Autodesk Inventor part; units mm, degrees
ref_plane "YZ Plane" through (0, 0, 0) normal (1, 0, 0) x (0, 1, 0)
ref_plane "XZ Plane" through (0, 0, 0) normal (0, 1, 0) x (-1, 0, 0)
ref_plane "XY Plane" through (0, 0, 0) normal (0, 0, 1) x (1, 0, 0)
sketch "Sketch1" plane through (0, 0, 0) normal (0, 0, 1) x (1, 0, 0)
  line L0 (0, 27) -> (138, 27)
  line L1 (138, 27) -> (138, 0)
  line L2 (138, 0) -> (138, -27)
  line L3 (138, -27) -> (27, -93) construction
  line L4 (27, -93) -> (0, -93)
  line L5 (0, -93) -> (0, 27) construction
  line L6 (0, 0) -> (138, 0) construction
  line L7 (0, 27) -> (-138, 27)
  line L8 (-138, 27) -> (-138, 0)
  line L9 (-138, 0) -> (-138, -27)
  line L10 (-138, -27) -> (-27, -93) construction
  line L11 (-27, -93) -> (0, -93)
  line L12 (27, -93) -> (138, -93)
  line L13 (138, -93) -> (138, -27)
  line L14 (-27, -93) -> (-138, -93)
  line L15 (-138, -93) -> (-138, -27)
  dimension "d0" = 138
  dimension "d2" = 27
  dimension "d3" = 54
  dimension "d4" = 27
  dimension "d5" = 120
extrude "Extrusion1" add sketch "Sketch1" along normal mid plane 60
sketch "Sketch2" plane through (-27, -93, 30) normal (0, -1, 0) x (1, 0, 0)
  circle A0 centre (27, -30) radius 24.5
  dimension "d20" = 49
extrude "Extrusion2" add sketch "Sketch2" along normal blind 51
sketch "Sketch3" plane through (-138, 27, 30) normal (0, 1, 0) x (1, 0, 0)
  circle A0 centre (138, 30) radius 10
  dimension "d12" = 20
extrude "Extrusion3" cut sketch "Sketch3" against normal through all
sketch "Sketch4" plane through (138, -27, 30) normal (1, 0, 0) x (0, 0, -1)
  circle A0 centre (30, 27) radius 10
  dimension "d16" = 20
extrude "Extrusion4" cut sketch "Sketch4" against normal through all
move or copy body "Move Body1" bodies to move or copy 1 copy no rotation origin (0, 0, 0) rotation axis (1, 0, 0) rotation angle 90
move or copy body "Move Body2" bodies to move or copy 1 copy no rotation origin (0, 0, 0) rotation axis (0, 0, 1) rotation angle 90
move or copy body "Move Body4" bodies to move or copy 1 copy no translate (0, 0, 144)
properties part number "UpperTorso_v2"
Input: part model. Units: mm. Frame: model coordinates. A direction names the side the tool comes from. Coordinates: 2 decimals unless noted, no trailing zeros. Write each loop counter-clockwise with the first axis right and the second up, starting at its lowest first coordinate (ties: lowest second). Pieces come first, ordered by that corner, then holes. Notation, with made-up numbers: (-34, 36) - (-7, 36) arc R15 cw to (-7, 57) - close; hole circle Ø4 at (-29, -30.75). An arc over 180 degrees is marked (long way). Put each result on its own line as item: value. Start each with the question number.
1) Ray query, L1, parallel to X at y = 0, z = 79; L2, parallel to Y at x = 0, z = 161.5; L3, parallel to Z at x = 0, y = -96. Return the intervals inside material, ascending.
2) Cut plane A-A (x = 0). Return the cut outline in (y, z).
3) Mould query, pull axis Z, two halves, no side actions, for faces 1 (the face through (30, -2, 112)), 2 (the face through (0, 11, 0)), 3 (the face through (2.17, -68.03, 134.24)). Classes: pulls with the +Z half, pulls with the -Z half, needs draft (parallel to the pull), parting line crosses it, or undercut.
4) Cut plane C-C (z = 76.5). Return the cut outline in (x, y), plus the area to 3 significant figures.
5) Cut plane D-D (x = 14). Return the cut outline in (y, z).
6) Reachability of faces 4 (the face through (-9.915, -1.302, 160.689)), 5 (the face through (-20.66, 13.17, 25.86)) from +Z, -Z, +X, -X, +Y, -Y: full face, straight path, thin tool, end or side. Return the list, or none.
7) Contact query for flat-ended pins moving along their axis: pin 1 (5 mm diameter, centred on x = 22.5, z = 33, fed in from -Y); pin 2 (16 mm diameter, centred on x = 0, y = 0, fed in from -Z); pin 3 (12 mm diameter, centred on y = -19.5, z = 28, fed in from -X); pin 4 (5 mm diameter, centred on x = 15, y = 91.5, fed in from -Z). Output: stop coordinate, or through.
8) Cut plane B-B (y = 39.5). Return the cut outline in (x, z).
Resolved:
1. L1: x = -30 to -10, 10 to 30
1. L2: y = -138 to -10, 10 to 138
1. L3: z = 51 to 134, 154 to 171
2. outline: (-138, 51) - (-24.5, 51) - (-24.5, 0) - (-10, 0) - (-10, 134) - (-138, 134) - close; (-138, 154) - (-10, 154) - (-10, 171) - (-138, 171) - close; (10, 0) - (24.5, 0) - (24.5, 51) - (138, 51) - (138, 134) - (10, 134) - close; (10, 154) - (138, 154) - (138, 171) - (10, 171) - close
3. face 1: needs draft
3. face 2: pulls with the -Z half
3. face 3: undercut
4. outline: (-30, -138) - (30, -138) - (30, 138) - (-30, 138) - close; hole circle Ø20 at (0, 0)
4. area: 16,200 mm2
5. outline: (-138, 51) - (-20.11, 51) - (-20.11, 0) - (20.11, 0) - (20.11, 51) - (138, 51) - (138, 171) - (-138, 171) - close
6. face 4: +Z, -Z
6. face 5: -Z
7. pin 1: stops at y = -14.15
7. pin 2: passes through
7. pin 3: stops at x = -20.45
7. pin 4: stops at z = 51
8. outline: (-30, 51) - (30, 51) - (30, 171) - (-30, 171) - close; hole circle Ø20 at (0, 144)
